from build123d import *

# Parameters (mm, degrees)
SKETCH_1_W           = 45
SKETCH_1_H           = 45
EXTRUDE_1_DEPTH      = 100
SKETCH_2_OUTSIDE_W   = 125.706
SKETCH_2_OUTSIDE_H   = 70.706
SKETCH_2_OUTSIDE_W_2 = 62
SKETCH_2_OUTSIDE_H_2 = 8
CUT_EXTRUDE_1_DEPTH  = 30
SKETCH_3_W           = 41
SKETCH_3_H           = 20.3
CUT_EXTRUDE_2_DEPTH  = 30.5
SKETCH_5_W           = 11.5
SKETCH_5_H           = 6.5
CUT_EXTRUDE_3_DEPTH  = 101
SKETCH_7_R           = 2.25
SKETCH_7_W           = 7
SKETCH_7_H           = 2
CUT_EXTRUDE_5_DEPTH  = 10
SKETCH_9_W           = 62
SKETCH_9_H           = 8
CUT_EXTRUDE_7_DEPTH  = 3
SKETCH_10_W          = 15
SKETCH_10_H          = 45
CUT_EXTRUDE_8_DEPTH  = 24
SKETCH_13_W          = 14
SKETCH_13_H          = 45
EXTRUDE_3_DEPTH      = 50
SKETCH_14_R          = 4.15
CUT_EXTRUDE_9_DEPTH  = 66
SKETCH_15_W          = 12
SKETCH_15_H          = 45
EXTRUDE_4_DEPTH      = 8
SKETCH_17_R          = 4.15
CUT_EXTRUDE_11_DEPTH = 46
SKETCH_8_W           = 35
SKETCH_8_H           = 10
CUT_EXTRUDE_12_DEPTH = 5
CUT_EXTRUDE_14_DEPTH = 1


with BuildPart() as part:
    # 草图1 → 凸台-拉伸1 (new body)
    with BuildSketch(Plane(origin=(0, 0, 0), x_dir=(0, 0, -1), z_dir=(1, 0, 0))):
        with Locations((-1.383662758, -144.856597142)):
            Rectangle(SKETCH_1_W, SKETCH_1_H)
    extrude(amount=EXTRUDE_1_DEPTH)

    # 草图2 outside → 切除-拉伸1 (cut)
    with BuildSketch(Plane(origin=(0, 0, -21.116337242), x_dir=(-1, 0, 0), z_dir=(0, 0, -1))):
        with Locations((-50, -144.857)):
            Rectangle(SKETCH_2_OUTSIDE_W, SKETCH_2_OUTSIDE_H)
        with Locations((-45, -141.856597142)):
            Rectangle(SKETCH_2_OUTSIDE_W_2, SKETCH_2_OUTSIDE_H_2, mode=Mode.SUBTRACT)
    extrude(amount=-CUT_EXTRUDE_1_DEPTH, mode=Mode.SUBTRACT)

    # 草图3 → 切除-拉伸2 (cut, through all)
    with BuildSketch(Plane(origin=(0, -137.856597142, 0), x_dir=(1, 0, 0), z_dir=(0, 1, 0))):
        with Locations((45.5, 3.766337242)):
            Rectangle(SKETCH_3_W, SKETCH_3_H)
    extrude(amount=-CUT_EXTRUDE_2_DEPTH, mode=Mode.SUBTRACT)

    # 草图5 → 切除-拉伸3 (cut, through all)
    with BuildSketch(Plane.ZY):
        with Locations((16.133662758, -128.606597142)):
            Rectangle(SKETCH_5_W, SKETCH_5_H)
        with Locations((16.133662758, -158.606597142)):
            Rectangle(SKETCH_5_W, SKETCH_5_H)
    extrude(amount=-CUT_EXTRUDE_3_DEPTH, mode=Mode.SUBTRACT)

    # 草图7 → 切除-拉伸5 (cut)
    with BuildSketch(Plane.XZ.offset(145.856597142)):
        with Locations((21.15, -8.916337242)):
            Circle(SKETCH_7_R)
        with Locations((21.15, 1.083662758)):
            Circle(SKETCH_7_R)
        with Locations((69.95, -8.916337242)):
            Circle(SKETCH_7_R)
        with Locations((69.95, 1.083662758)):
            Circle(SKETCH_7_R)
        with Locations((21.5, -3.916337242)):
            Rectangle(SKETCH_7_W, SKETCH_7_H)
        with Locations((69.5, -3.916337242)):
            Rectangle(SKETCH_7_W, SKETCH_7_H)
    extrude(amount=-CUT_EXTRUDE_5_DEPTH, mode=Mode.SUBTRACT)

    # 草图9 → 切除-拉伸7 (cut)
    with BuildSketch(Plane(origin=(0, 0, -21.116337242), x_dir=(-1, 0, 0), z_dir=(0, 0, -1))):
        with Locations((-45, -141.856597142)):
            Rectangle(SKETCH_9_W, SKETCH_9_H)
    extrude(amount=-CUT_EXTRUDE_7_DEPTH, mode=Mode.SUBTRACT)

    # 草图10 → 切除-拉伸8 (cut)
    with BuildSketch(Plane(origin=(100, 0, 0), x_dir=(0, 0, -1), z_dir=(1, 0, 0))):
        with Locations((-16.383662758, -144.856597142)):
            Rectangle(SKETCH_10_W, SKETCH_10_H)
    extrude(amount=-CUT_EXTRUDE_8_DEPTH, mode=Mode.SUBTRACT)

    # 草图13 → 凸台-拉伸3 (add)
    with BuildSketch(Plane(origin=(0, 0, 8.883662758), x_dir=(-1, 0, 0), z_dir=(0, 0, -1))):
        with Locations((-7, -144.856597142)):
            Rectangle(SKETCH_13_W, SKETCH_13_H)
    extrude(amount=EXTRUDE_3_DEPTH)

    # 草图14 → 切除-拉伸9 (cut, through all)
    with BuildSketch(Plane(origin=(0, 0, -41.116337242), x_dir=(-1, 0, 0), z_dir=(0, 0, -1))):
        with Locations((-7, -142.356597142)):
            Circle(SKETCH_14_R)
    extrude(amount=-CUT_EXTRUDE_9_DEPTH, mode=Mode.SUBTRACT)

    # 草图15 → 凸台-拉伸4 (add)
    with BuildSketch(Plane(origin=(14, 0, 0), x_dir=(0, 0, -1), z_dir=(1, 0, 0))):
        with Locations((18.668900169, -144.856597142)):
            Rectangle(SKETCH_15_W, SKETCH_15_H)
    extrude(amount=EXTRUDE_4_DEPTH)

    # 草图17 → 切除-拉伸11 (cut, through all)
    with BuildSketch(Plane.XZ.offset(167.356597142)):
        with Locations((17, -18.616337242)):
            Circle(SKETCH_17_R)
    extrude(amount=-CUT_EXTRUDE_11_DEPTH, mode=Mode.SUBTRACT)

    # 草图8 → 切除-拉伸12 (cut)
    with BuildSketch(Plane(origin=(0, 0, 8.883662758), x_dir=(-1, 0, 0), z_dir=(0, 0, -1))):
        with Locations((-54.391773718, -128.856597142)):
            Rectangle(SKETCH_8_W, SKETCH_8_H)
    extrude(amount=-CUT_EXTRUDE_12_DEPTH, mode=Mode.SUBTRACT)

    # 草图18 → 切除-拉伸14 (cut)
    with BuildSketch(Plane.XZ.offset(145.856597142)):
        Polygon((76, 8.883662758), (22, 8.883662758), (14, 8.883662758), (14, -12.654298783), (22, -12.654298783), (22, -18.116337242), (76, -18.116337242), align=None)
    extrude(amount=-CUT_EXTRUDE_14_DEPTH, mode=Mode.SUBTRACT)


solid = part.part
The model under review builds one solid part; all positions refer to its coordinate system, in mm. A direction names the side the tool comes from. Coordinates: 2 decimals unless noted, no trailing zeros. Loops run counter-clockwise (first coordinate to the right, second up) from the corner with the lowest first, then second, coordinate; pieces in that order, holes last. Notation, with made-up numbers: M -16.5,-5 L -9.5,-5 A24 cw -9.5,19 Z; hole C 70.25,-30 d1. An arc over 180 degrees is marked long. Put each result on its own line as item: value. Start each with the question number.
Q1. Add section B-B (x = 32). Write out the cut boundary in (y, z), and give its area (3 significant figures).
Q2. Clearance check with flat-ended pins moving along their axes: pin 1 (3 mm diameter, centred on y = -161.5, z = -18.5, fed in from -X); pin 2 (13 mm diameter, centred on y = -143.5, z = -31, fed in from +X); pin 3 (5.5 mm diameter, centred on x = 56, y = -139.5, fed in from -Z); pin 4 (1.2 mm diameter, centred on x = 47, y = -125, fed in from -Z). State where each tip first meets the part, or that it passes through.
Q3. Add section D-D (z = -17). Write out the cut boundary in (x, y).
Q4. For faces 5 (the flat face through (18, -157, -12.669)), 6 (the flat face through (37, -145, 23.884)), 7 (the flat face through (37, -159, 10.384)), 8 (the cylindrical face through (7.9, -146.408, -9.071)), 9 (the flat face through (66, -141, -9)), list the 3-axis set-ups (+Z, -Z, +X, -X, +Y, -Y) from which the entire face can be reached by the end or side of a thin tool; tool diameter is ignored.
Q5. The part is to be moulded in two halves that separate along X. For faces 1 (the flat face through (36.892, -129, 10)), 2 (the flat face through (14, -130, -2)), 3 (the flat face through (55, -133, 13.884)), 4 (the flat face through (12, -145, -41.116)), say which applies: +X half, -X half, draft (parallel to the pull), parting line (faces both ways), or undercut.
Q6. Add section A-A (x = 69.95). Count the separate pieces of the cut face and the enclosed holes in it, and give its area (3 significant figures).
Q7. Wall thickness on line 1 (Y direction, x = 73, z = 11); line 2 (Z direction, x = 17, y = -131.5); line 3 (X direction, y = -125.5, z = -18.5): over which ranges is each line inside the solid? List them lowest first.
Answers:
1. outline: M -167.36,8.88 L -144.86,8.88 L -144.86,6.38 L -137.86,6.38 L -137.86,8.88 L -122.36,8.88 L -122.36,23.88 L -167.36,23.88 Z; M -144.86,-18.12 L -137.86,-18.12 L -137.86,-13.92 L -144.86,-13.92 Z; hole M -161.86,10.38 L -155.36,10.38 L -155.36,21.88 L -161.86,21.88 Z; hole M -131.86,10.38 L -125.36,10.38 L -125.36,21.88 L -131.86,21.88 Z
1. area: 572 mm^2
2. pin 1: stops at x = 0
2. pin 2: stops at x = 22
2. pin 3: stops at z = -18.12
2. pin 4: stops at z = 13.88
3. outline: M 0,-167.36 L 13.18,-167.36 L 13.18,-122.36 L 0,-122.36 Z; M 20.82,-167.36 L 22,-167.36 L 22,-144.86 L 76,-144.86 L 76,-137.86 L 22,-137.86 L 22,-122.36 L 20.82,-122.36 Z; hole C 7,-142.36 d8.3
4. face 5: +X, -Y
4. face 6: +Z, +X, -X, +Y, -Y
4. face 7: +X, -X
4. face 8: +Z, -Z
4. face 9: +Y, -Y
5. face 1: undercut
5. face 2: +X half
5. face 3: undercut
5. face 4: draft
6. separate pieces: 4
6. enclosed holes: 1
6. area: 610 mm^2
7. line 1: y = -167.36 to -161.86, -155.36 to -131.86, -125.36 to -122.36
7. line 2: z = -24.67 to -22.77, -14.47 to -12.67, 8.88 to 10.38, 21.88 to 23.88
7. line 3: x = 0 to 12.85, 21.15 to 22
